Autodesk Inventor part; units mm, degrees
ref_plane "YZ Plane" through (0, 0, 0) normal (1, 0, 0) x (0, 1, 0)
ref_plane "XZ Plane" through (0, 0, 0) normal (0, 1, 0) x (-1, 0, 0)
ref_plane "XY Plane" through (0, 0, 0) normal (0, 0, 1) x (1, 0, 0)
sketch "Sketch1" plane through (0, 0, 0) normal (0, 1, 0) x (-1, 0, 0)
  circle A0 centre (0, 0) radius 3.5
  circle A1 centre (0, 0) radius 2.35
  dimension "d0" = 7
  dimension "d1" = 4.7
extrude "Extrusion1" add sketch "Sketch1" along normal blind 11 contours A1
extrude "Extrusion2" add sketch "Sketch1" along normal blind 2
sketch "Sketch2" plane through (0, 11, 0) normal (0, 1, 0) x (1, 0, 0)
  circle A0 centre (0, 0) radius 1.5
  dimension "d6" = 3
extrude "Extrusion3" cut sketch "Sketch2" against normal blind 7
properties part number "Locker1_3DPrint"
Here's how the part is built. I have some questions about the finished solid (model axes, mm). A direction names the side the tool comes from. Give positions to 0.01 mm unless a question says otherwise; leave off trailing zeros. Order: outer loops, then holes, each group sorted by start corner. A loop starts at its lowest first (then second) coordinate and runs counter-clockwise, first axis right, second up. Notation, with made-up numbers: (23, 56.5) - (80, 56.5) arc R11 cw to (80, 71.5) - close; hole circle Ø8 at (76.25, -2.75). An arc over 180 degrees is marked (long way). Answer as a JSON object with one key per item and string values. Group by question number.
Item 1: If we section it at D-D on y = 1.5: Please give me the cut outline in (x, z).
Item 2: If we section it at C-C on x = 0: Please give me the cut outline in (y, z), and give its area (3 significant figures).
Item 3: If we section it at A-A on y = 4.25: Please give me the cut outline in (x, z).
Item 4: Which directions (+Z, -Z, +X, -X, +Y, -Y) give clear straight access to the entire face, cutting with the end or side of a thin tool? Please do faces 1 (the flat face through (0, 4, 0)), 2 (the flat face through (0, 11, -2)).
Item 5: If we section it at B-B on z = 0: Please give me the cut outline in (x, y), and give its area (3 significant figures).
Item 6: If we mould it in two halves opening along Z, with no side actions, what happens to faces 3 (the flat face through (0, 0, 0)), 4 (the cylindrical face through (0.509, 6.437, 2.294)), 5 (the cylindrical face through (-1.5, 7.55, -0.07))? For each: pulls with the +Z half, pulls with the -Z half, needs draft (parallel to the pull), parting line crosses it, or undercut.
Item 7: For P1, Ø1.5, axis at y = 8.5, z = -2, coming from the +X side; P2, Ø1.5, axis at x = 0.5, z = 0, coming from the +Y side; P3, Ø2, axis at x = 0, y = 6.5, coming from the -Z side; P4, Ø2.5, axis at x = 0, z = 0, coming from the -Y side, each with a flat end and sliding along its axis, tell me the tip position at first contact or that it passes through.
Item 8: Please list where these lines run through material, in increasing order: probe 1 along Z at (x, y) = (0, 9); probe 2 along Y at (x, z) = (3, -0.75); probe 3 along Z at (x, y) = (1, 6).
Result set:
{
 "1": {"outline": "circle Ø7 at (0, 0)"},
 "2": {"outline": "(0, -3.5) - (2, -3.5) - (2, -2.35) - (11, -2.35) - (11, -1.5) - (4, -1.5) - (4, 1.5) - (11, 1.5) - (11, 2.35) - (2, 2.35) - (2, 3.5) - (0, 3.5) - close", "area": "35.3 mm²"},
 "3": {"outline": "circle Ø4.7 at (0, 0); hole circle Ø3 at (0, 0)"},
 "4": {"face 1": "+Y", "face 2": "+Z, -Z, +X, -X, +Y"},
 "5": {"outline": "(-3.5, 0) - (3.5, 0) - (3.5, 2) - (2.35, 2) - (2.35, 11) - (1.5, 11) - (1.5, 4) - (-1.5, 4) - (-1.5, 11) - (-2.35, 11) - (-2.35, 2) - (-3.5, 2) - close", "area": "35.3 mm²"},
 "6": {"face 3": "needs draft", "face 4": "parting line crosses it", "face 5": "undercut"},
 "7": {"P1": "x = 1.99", "P2": "y = 4", "P3": "z = -2.35", "P4": "y = 0"},
 "8": {"probe 1": "-2.35 to -1.5, 1.5 to 2.35", "probe 2": "0 to 2", "probe 3": "-2.13 to -1.12, 1.12 to 2.13"}
}
